Geometry check sheet. Reference: the model listing, model coordinates, mm. Face numbers are marked on the shaded views. Coordinates: 2 decimals unless noted, no trailing zeros.
from build123d import *

# Parameters (mm, degrees)
SKETCH1_R           = 21.717
SKETCH1_R_2         = 18.542
BOSS_EXTRUDE1_DEPTH = 355.6
CUT_SWEEP1_PITCH    = 152.4


with BuildPart() as part:
    # Sketch1 → Boss-Extrude1 (new body)
    with BuildSketch(Plane(origin=(0, 0, 0), x_dir=(1, 0, 0), z_dir=(0, 1, 0))):
        with Locations(Location((0, 0, 0), (0, 0, 270))):
            Circle(SKETCH1_R)
        with Locations(Location((0, 0, 0), (0, 0, 270))):
            Circle(SKETCH1_R_2, mode=Mode.SUBTRACT)
    extrude(amount=BOSS_EXTRUDE1_DEPTH)

    # Cut-Sweep1: the profile of Sketch6 profile screwed along a right-hand helix of 0.96 turns, 38 arcs to a turn; built about Z, then put on its axis
    cut_sweep1_z = Axis((0, 0, 0), (0, 0, 1))
    cut_sweep1_corners = [(18.542, 0, -22.86), (21.7173, 0, -22.86), (21.7173, 0, 22.86), (18.542, 0, 22.86)]
    with BuildLine(mode=Mode.PRIVATE) as cut_sweep1_profile:
        Line(cut_sweep1_corners[0], cut_sweep1_corners[1])
        Line(cut_sweep1_corners[1], cut_sweep1_corners[2])
        Line(cut_sweep1_corners[2], cut_sweep1_corners[3])
        Line(cut_sweep1_corners[3], cut_sweep1_corners[0])
    cut_sweep1_cap = Face(cut_sweep1_profile.wire())
    cut_sweep1_turn_angles = [0, 4.736842105, 9.473684211, 14.210526316, 18.947368421, 23.684210526, 28.421052632, 33.157894737, 37.894736842, 42.631578947, 47.368421053, 52.105263158, 56.842105263, 61.578947368, 66.315789474, 71.052631579, 75.789473684, 80.526315789, 85.263157895, 90, 94.736842105, 99.473684211, 104.210526316, 108.947368421, 113.684210526, 118.421052632, 123.157894737, 127.894736842, 132.631578947, 137.368421053, 142.105263158, 146.842105263, 151.578947368, 156.315789474, 161.052631579, 165.789473684, 170.526315789, 175.263157895, 180, 184.736842105, 189.473684211, 194.210526316, 198.947368421, 203.684210526, 208.421052632, 213.157894737, 217.894736842, 222.631578947, 227.368421053, 232.105263158, 236.842105263, 241.578947368, 246.315789474, 251.052631579, 255.789473684, 260.526315789, 265.263157895, 270, 274.736842105, 279.473684211, 284.210526316, 288.947368421, 293.684210526, 298.421052632, 303.157894737, 307.894736842, 312.631578947, 317.368421053, 322.105263158, 326.842105263, 331.578947368, 336.315789474, 341.052631579, 343.326315789, 345.6]
    cut_sweep1_turn_weights = [1, 0.9965844930066698, 1, 0.9965844930066698, 1, 0.9965844930066698, 1, 0.9965844930066698, 1, 0.9965844930066698, 1, 0.9965844930066698, 1, 0.9965844930066698, 1, 0.9965844930066698, 1, 0.9965844930066698, 1, 0.9965844930066698, 1, 0.9965844930066698, 1, 0.9965844930066698, 1, 0.9965844930066698, 1, 0.9965844930066698, 1, 0.9965844930066698, 1, 0.9965844930066698, 1, 0.9965844930066698, 1, 0.9965844930066698, 1, 0.9965844930066698, 1, 0.9965844930066698, 1, 0.9965844930066698, 1, 0.9965844930066698, 1, 0.9965844930066698, 1, 0.9965844930066698, 1, 0.9965844930066698, 1, 0.9965844930066698, 1, 0.9965844930066698, 1, 0.9965844930066698, 1, 0.9965844930066698, 1, 0.9965844930066698, 1, 0.9965844930066698, 1, 0.9965844930066698, 1, 0.9965844930066698, 1, 0.9965844930066698, 1, 0.9965844930066698, 1, 0.9965844930066698, 1, 0.9992127221406268, 1]
    cut_sweep1_turn_rails = [Edge.make_bspline([Vector(p[0], p[1], 0).rotate(cut_sweep1_z, cut_sweep1_turn_angles[k]) / cut_sweep1_turn_weights[k] + Vector(0, 0, p[2] + CUT_SWEEP1_PITCH * cut_sweep1_turn_angles[k] / 360) for k in range(75)], [0, 0, 0, 1, 1, 2, 2, 3, 3, 4, 4, 5, 5, 6, 6, 7, 7, 8, 8, 9, 9, 10, 10, 11, 11, 12, 12, 13, 13, 14, 14, 15, 15, 16, 16, 17, 17, 18, 18, 19, 19, 20, 20, 21, 21, 22, 22, 23, 23, 24, 24, 25, 25, 26, 26, 27, 27, 28, 28, 29, 29, 30, 30, 31, 31, 32, 32, 33, 33, 34, 34, 35, 35, 36, 36, 37, 37, 37], 2, cut_sweep1_turn_weights) for p in cut_sweep1_corners]
    cut_sweep1_turn_sides = [Face.make_surface_from_curves(cut_sweep1_turn_rails[p[0]], cut_sweep1_turn_rails[p[1]]) for p in [(0, 1), (1, 2), (2, 3), (3, 0)]]
    cut_sweep1 = Plane(origin=(0, 182.88, 0), x_dir=(0, 0, 1), z_dir=(0, 1, 0)) * Solid(Shell([*cut_sweep1_turn_sides, cut_sweep1_cap, cut_sweep1_cap.rotate(cut_sweep1_z, 345.6).moved(Location((0, 0, CUT_SWEEP1_PITCH * 345.6 / 360)))]))
    add(cut_sweep1, mode=Mode.SUBTRACT)


solid = part.part
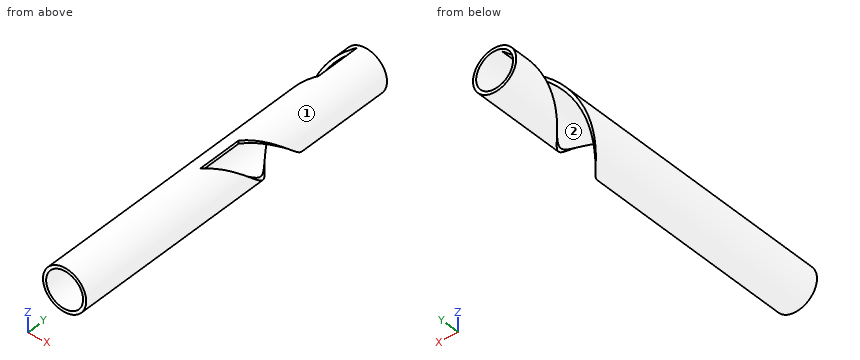
(1) Scan lines: L1, parallel to X at y = 126, z = 0; L2, parallel to Z at x = 11, y = 142. Record each from-to range of solid material in increasing order.
Findings:
L1: x = -21.72 to -18.54, 18.54 to 21.72
L2: z = -18.73 to -14.93, 14.93 to 18.73
(2) Sectioned sample at A-A on z = 0. State how many separate pieces and enclosed holes the cut face has, and give its area (3 significant figures).
Findings:
separate pieces: 4
enclosed holes: 0
area: 1,970 mm2
(3) Gauge pin test, flat ends, axial feed: pin 1 Ø1.5 at (x, y) = (13.5, 77.5) entering from -Z; pin 2 Ø1 at (y, z) = (193, 19.5) entering from +X; pin 3 Ø5 at (x, z) = (12, 6.5) entering from -Y; pin 4 Ø12 at (y, z) = (285.5, -10.5) entering from +X. Record the tip position at first contact, or that the pin passes through.
Findings:
pin 1: stops at z = -17.58
pin 2: stops at x = 0
pin 3: passes through
pin 4: stops at x = 21.25
(4) Draft check along X on the marked faces 1 and 2. Enter one of: +X half, -X half, draft (parallel to the pull), parting line (faces both ways), or undercut.
Findings:
face 1: parting line
face 2: undercut
